Source: CAD feature listing. Evaluate the final solid. Frame: model axes, mm. Give positions to 0.01 mm unless a question says otherwise; leave off trailing zeros. Write each loop counter-clockwise with the first axis right and the second up, starting at its lowest first coordinate (ties: lowest second). Pieces come first, ordered by that corner, then holes. Notation, with made-up numbers: M 45.5,44.25 L 96.5,44.25 A17 ccw 96.5,65.25 Z; hole C 2,75 d11. An arc over 180 degrees is marked long. Return JSON: item names as keys, results as strings.
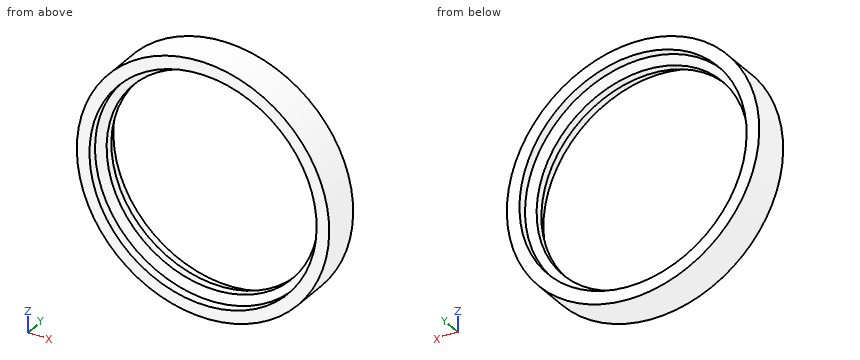
```python
from build123d import *

# Parameters (mm, degrees)
CROQUIS1_R              = 50
CROQUIS1_R_2            = 42
SALIENTE_EXTRUIR1_DEPTH = 15


with BuildPart() as part:
    # Croquis1 → Saliente-Extruir1 (new body)
    with BuildSketch(Plane(origin=(0, 0, 0), x_dir=(1, 0, 0), z_dir=(0, 1, 0))):
        with Locations(Location((0, 0, 0), (0, 0, 270))):
            Circle(CROQUIS1_R)
        with Locations(Location((0, 0, 0), (0, 0, 270))):
            Circle(CROQUIS1_R_2, mode=Mode.SUBTRACT)
    extrude(amount=SALIENTE_EXTRUIR1_DEPTH)

    # Croquis3 → Cortar-Revolución1 (revolve, cut)
    with BuildSketch(Plane.XY, mode=Mode.PRIVATE) as cortar_revoluci_n1_sk:
        Polygon((-45, 11.517298894), (-42, 9), (-42, 15), (-45, 15), align=None)
        Polygon((-45, 0), (-42, 0), (-42, 6), (-45, 3.482701106), align=None)
    revolve(cortar_revoluci_n1_sk.sketch.rotate(Axis((0, 3.82587886, 0), (0, -1, 0)), 270), axis=Axis((0, 3.82587886, 0), (0, -1, 0)), mode=Mode.SUBTRACT)


solid = part.part
```
1) Contact query for flat-ended pins moving along their axis: pin 1 Ø5 at (y, z) = (6.5, -21) entering from +X; pin 2 Ø4 at (y, z) = (9.5, -23.5) entering from +X; pin 3 Ø6 at (x, z) = (29, -33.5) entering from -Y; pin 4 Ø5 at (y, z) = (6, -30) entering from -X. Output: stop coordinate, or through.
Numbers:
{"pin 1": "stops at x = 46.45", "pin 2": "stops at x = 45.14", "pin 3": "stops at y = 0", "pin 4": "stops at x = -41.76"}
2) Cut plane A-A, the plane z = 0. Return the cut outline in (x, y), then the cut area to 3 significant figures.
Numbers:
{"outline": "M -50,0 L -45,0 L -45,3.48 L -42,6 L -42,9 L -45,11.52 L -45,15 L -50,15 Z; M 42,6 L 45,3.48 L 45,0 L 50,0 L 50,15 L 45,15 L 45,11.52 L 42,9 Z", "area": "183 mm²"}
3) Line query: line 1 (X direction, y = 1.95, z = 0); line 2 (Z direction, x = -9, y = 14); line 3 (Z direction, x = 5.5, y = 4). Output: solid intervals per line, ascending. Write a range as [from, to].
Numbers:
{"line 1": "x = [-50, -45], [45, 50]", "line 2": "z = [-49.18, -44.09], [44.09, 49.18]", "line 3": "z = [-49.7, -44.04], [44.04, 49.7]"}
4) Cut plane B-B, the plane x = 0. Return the cut outline in (y, z), then the cut area to 3 significant figures.
Numbers:
{"outline": "M 0,-50 L 15,-50 L 15,-45 L 11.52,-45 L 9,-42 L 6,-42 L 3.48,-45 L 0,-45 Z; M 0,45 L 3.48,45 L 6,42 L 9,42 L 11.52,45 L 15,45 L 15,50 L 0,50 Z", "area": "183 mm²"}
